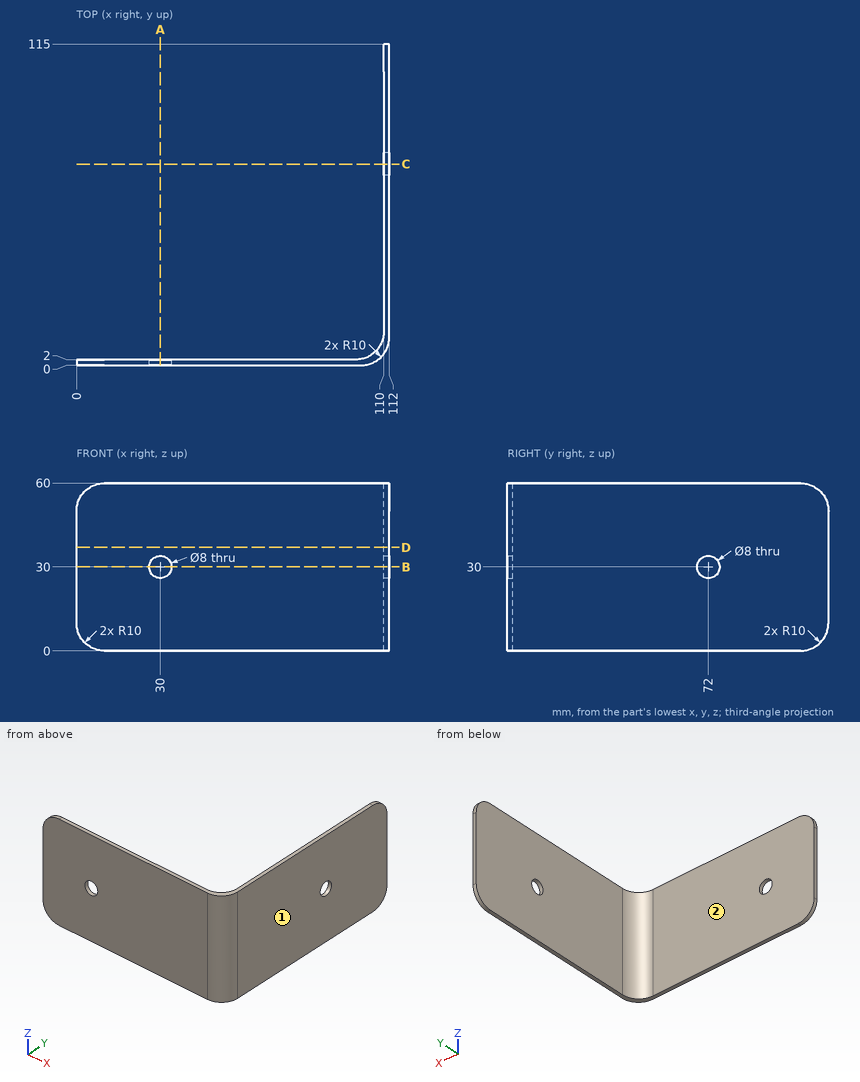
Can you work these out from the drawing? Everything is in mm from the part's minimum corner. A direction names the side the tool comes from. Coordinates: 2 decimals unless noted, no trailing zeros. Write each loop counter-clockwise with the first axis right and the second up, starting at its lowest first coordinate (ties: lowest second). Pieces come first, ordered by that corner, then holes. Notation, with made-up numbers: (81, 68.5) - (126, 68.5) arc R13 cw to (126, 74.5) - close; hole circle Ø4 at (76, 88). An arc over 180 degrees is marked (long way). Use a Markdown table: item, result.
Q1. I'm going to push flat-ended pins straight in: pin 1 Ø1.5 at (y, z) = (47.5, 53) entering from -X; pin 2 Ø8 at (x, z) = (85.5, 27.5) entering from +Y. Where does each tip first touch, or does it pass through?
Geometry check:
| item | result |
|---|---|
| pin 1 | stops at x = 110 |
| pin 2 | stops at y = 2 |
Q2. Imagine slicing it at A-A (x = 30). List the corners of the cut face in (y, z) for me.
Geometry check:
| item | result |
|---|---|
| outline | (0, 0) - (2, 0) - (2, 26) - (0, 26) - close; (0, 34) - (2, 34) - (2, 60) - (0, 60) - close |
Q3. Which directions (+Z, -Z, +X, -X, +Y, -Y) give clear straight access to the entire face, cutting with the end or side of a thin tool? Please do the marked faces 1 and 2.
Geometry check:
| item | result |
|---|---|
| face 1 | +Z, -Z, +X, +Y, -Y |
| face 2 | +Z, -Z, -X, +Y |
Q4. Imagine slicing it at C-C (y = 72). List the corners of the cut face in (x, z) for me, and give its area (3 significant figures).
Geometry check:
| item | result |
|---|---|
| outline | (110, 0) - (112, 0) - (112, 26) - (110, 26) - close; (110, 34) - (112, 34) - (112, 60) - (110, 60) - close |
| area | 104 mm2 |
Q5. Imagine slicing it at B-B (z = 30). List the corners of the cut face in (x, y) for me, and give its area (3 significant figures).
Geometry check:
| item | result |
|---|---|
| outline | (0, 0) - (26, 0) - (26, 2) - (0, 2) - close; (34, 0) - (102, 0) arc R10 ccw to (112, 10) - (112, 68) - (110, 68) - (110, 12) arc R10 cw to (100, 2) - (34, 2) - close; (110, 76) - (112, 76) - (112, 115) - (110, 115) - close |
| area | 418 mm2 |
Q6. Please list where these lines run through material, in increasing order: L1, parallel to Z at x = 30, y = 1; L2, parallel to X at y = 20.5, z = 8.5; L3, parallel to Y at x = 91, z = 31.5.
Geometry check:
| item | result |
|---|---|
| L1 | z = 0 to 26, 34 to 60 |
| L2 | x = 110 to 112 |
| L3 | y = 0 to 2 |
Q7. Imagine slicing it at D-D (z = 37). List the corners of the cut face in (x, y) for me.
Geometry check:
| item | result |
|---|---|
| outline | (0, 0) - (102, 0) arc R10 ccw to (112, 10) - (112, 115) - (110, 115) - (110, 12) arc R10 cw to (100, 2) - (0, 2) - close |
